Source: CAD feature listing. Evaluate the final solid. Frame: model axes, mm. Face numbers are marked on the shaded views. Give positions to 0.01 mm unless a question says otherwise; leave off trailing zeros. Write each loop counter-clockwise with the first axis right and the second up, starting at its lowest first coordinate (ties: lowest second). Pieces come first, ordered by that corner, then holes. Notation, with made-up numbers: (-5.75, 34) -> (-0.75, 34) arc R25 cw to (-0.75, 66) -> close; hole circle Ø6 at (-17, 12.5). An arc over 180 degrees is marked (long way). Answer as a JSON object with one key per item and string values. Group by question number.
Item 1: Section query C-C on x = 44. Return the cut outline in (y, z), plus the area to 3 significant figures.
Item 2: Section query A-A on x = 72.5. Return the cut outline in (y, z).
Item 3: Section query D-D on y = 18. Return the cut outline in (x, z), plus the area to 3 significant figures.
Item 4: First-contact query: pin 1 Ø3 at (y, z) = (-30.5, 1) entering from -X; pin 2 Ø1.4 at (x, z) = (-89.5, 1) entering from +Y; pin 3 Ø1.4 at (y, z) = (30, 1) entering from +X; pin 4 Ø0.9 at (y, z) = (-31.5, 1) entering from +X. Flat tips, straight axial feed; report the tip coordinate or a pass-through.
Item 5: Pull-direction query (X, two-part tool) for the marked faces 1 and 2; classes: pulls with the +X half, pulls with the -X half, needs draft (parallel to the pull), parting line crosses it, or undercut.
Item 6: Section query B-B on y = -10. Give the number of separate pieces and of enclosed holes in the cut face, plus the area to 3 significant figures.
Item 7: Ray query, probe 1 along X at (y, z) = (-6, 10); probe 2 along X at (y, z) = (-6, 2.75); probe 3 along Y at (x, z) = (44, 10). Return the intervals inside material, ascending. Write a range as from..to.
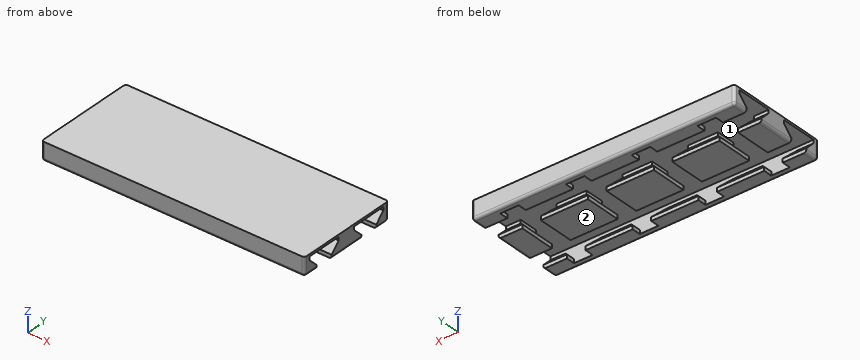
from build123d import *

# Parameters (mm, degrees)
SKETCH1_W           = 77
SKETCH1_H           = 196
BOSS_EXTRUDE1_DEPTH = 13.5
CUT_EXTRUDE1_DEPTH  = 201.201148848
CUT_EXTRUDE2_START  = -72.4
CUT_EXTRUDE2_DEPTH  = 67.8
FILLET1_R           = 2


with BuildPart() as part:
    # Sketch1 → Boss-Extrude1 (new body)
    with BuildSketch(Plane(origin=(0, 0, 0), x_dir=(0, 1, 0), z_dir=(0, 0, 1))):
        Rectangle(SKETCH1_W, SKETCH1_H)
    extrude(amount=BOSS_EXTRUDE1_DEPTH)

    # Sketch2 → Cut-Extrude1 (cut, through all)
    with BuildSketch(Plane(origin=(-98, 0, 0), x_dir=(0, -1, 0), z_dir=(-1, 0, 0))):
        Polygon((13.6, 2.834314575), (13.6, 0), (27.4, 0), (27.4, 2.834314575), (33.9, 9.334314575), (33.9, 11.9), (7.1, 11.9), (7.1, 9.334314575), align=None)
        Polygon((-27.4, 2.834314575), (-27.4, 0), (-13.6, 0), (-13.6, 2.834314575), (-7.1, 9.334314575), (-7.1, 11.9), (-33.9, 11.9), (-33.9, 9.334314575), align=None)
    extrude(amount=-CUT_EXTRUDE1_DEPTH, mode=Mode.SUBTRACT)

    # Sketch3 → Cut-Extrude2 (cut)
    with BuildSketch(Plane.XZ.offset(38.5).offset(CUT_EXTRUDE2_START)):
        Polygon((-80.4, 2.834314575), (-80.4, 0), (-66.6, 0), (-66.6, 2.834314575), (-60.1, 9.334314575), (-60.1, 11.9), (-86.9, 11.9), (-86.9, 9.334314575), align=None)
        Polygon((-31.4, 2.834314575), (-31.4, 0), (-17.6, 0), (-17.6, 2.834314575), (-11.1, 9.334314575), (-11.1, 11.9), (-37.9, 11.9), (-37.9, 9.334314575), align=None)
        Polygon((17.6, 2.834314575), (17.6, 0), (31.4, 0), (31.4, 2.834314575), (37.9, 9.334314575), (37.9, 11.9), (11.1, 11.9), (11.1, 9.334314575), align=None)
        Polygon((66.6, 0), (80.4, 0), (80.4, 2.834314575), (86.9, 9.334314575), (86.9, 11.9), (60.1, 11.9), (60.1, 9.334314575), (66.6, 2.834314575), align=None)
    extrude(amount=CUT_EXTRUDE2_DEPTH, mode=Mode.SUBTRACT)

    # Fillet1
    fillet1_edges = [part.edges().sort_by_distance(p)[0] for p in [
        (98, 0, 0),
        (98, 32.95, 0),
        (-98, 0, 0),
        (-98, -32.95, 0),
        (98, -32.95, 0),
        (0, -38.5, 0),
        (-98, 32.95, 0),
        (0, 38.5, 0),
        (98, 38.5, 6.75),
        (98, -38.5, 6.75),
        (-98, -38.5, 6.75),
        (-98, 38.5, 6.75),
    ]]
    fillet(fillet1_edges, radius=FILLET1_R)


solid = part.part
Worked answers:
{
 "1": {"outline": "(-38.5, 2) arc R2 ccw to (-36.5, 0) -> (-27.4, 0) -> (-27.4, 2.83) -> (-33.9, 9.33) -> (-33.9, 11.9) -> (-7.1, 11.9) -> (-7.1, 9.33) -> (-13.6, 2.83) -> (-13.6, 0) -> (13.6, 0) -> (13.6, 2.83) -> (7.1, 9.33) -> (7.1, 11.9) -> (33.9, 11.9) -> (33.9, 9.33) -> (27.4, 2.83) -> (27.4, 0) -> (36.5, 0) arc R2 ccw to (38.5, 2) -> (38.5, 13.5) -> (-38.5, 13.5) -> close", "area": "558 mm^2"},
 "2": {"outline": "(-38.5, 2) arc R2 ccw to (-36.5, 0) -> (-33.9, 0) -> (-33.9, 11.9) -> (33.9, 11.9) -> (33.9, 0) -> (36.5, 0) arc R2 ccw to (38.5, 2) -> (38.5, 13.5) -> (-38.5, 13.5) -> close"},
 "3": {"outline": "(-98, 11.9) -> (98, 11.9) -> (98, 13.5) -> (-98, 13.5) -> close", "area": "314 mm^2"},
 "4": {"pin 1": "x = -98", "pin 2": "y = 38.48", "pin 3": "x = 97.98", "pin 4": "x = 97.92"},
 "5": {"face 1": "undercut", "face 2": "needs draft"},
 "6": {"separate pieces": "6", "enclosed holes": "0", "area": "1,170 mm^2"},
 "7": {"probe 1": "-98..-86.9, -60.1..-37.9, -11.1..11.1, 37.9..60.1, 86.9..98", "probe 2": "-98..-80.4, -66.6..-31.4, -17.6..17.6, 31.4..66.6, 80.4..98", "probe 3": "-38.5..-33.9, -7.1..7.1, 33.9..38.5"}
}
